from build123d import *

# Parameters (mm, degrees)
F0_W      = 64
F0_H      = 76
F1_DEPTH  = 72
F2_T      = -13
F3_R      = 12.5
F4_DEPTH  = 100
F5_W      = 76
F5_H      = 18
F6_DEPTH  = 56
F8_DEPTH  = 25
F9_W      = 22
F9_H      = 54
F10_DEPTH = 52
F12_DEPTH = 25


with BuildPart() as f1:
    # F0 (on Top) → F1 (new body)
    with BuildSketch(Plane.XY):
        with Locations((32, 38)):
            Rectangle(F0_W, F0_H)
    extrude(amount=F1_DEPTH)

    # F2
    f2_openings = [f1.faces().sort_by_distance(p)[0] for p in [
        (32, 38, 72),
    ]]
    offset(amount=F2_T, openings=f2_openings)

    # F3 (on face) → F4 (cut)
    with BuildSketch(Plane.XZ):
        with Locations((32, 36)):
            Circle(F3_R)
    extrude(amount=-F4_DEPTH, mode=Mode.SUBTRACT)

    # F5 (on face) → F6 (join)
    with BuildSketch(Plane(origin=(0, 0, 0), x_dir=(0, -1, 0), z_dir=(-1, 0, 0))):
        with Locations((-38, 9)):
            Rectangle(F5_W, F5_H)
    extrude(amount=F6_DEPTH)

    # F7 (on face) → F8 (cut)
    with BuildSketch(Plane.XY.offset(18)):
        with BuildLine():
            ThreePointArc((-56, 38), (-44.870058, 64.870058), (-18, 76))
            Line((-18, 76), (-56, 76))
            Line((-56, 76), (-56, 38))
        make_face()
        with BuildLine():
            ThreePointArc((-18, 0), (-44.870058, 11.129942), (-56, 38))
            Line((-56, 38), (-56, 0))
            Line((-56, 0), (-18, 0))
        make_face()
    extrude(amount=-F8_DEPTH, mode=Mode.SUBTRACT)

    # F9 (on face) → F10 (join)
    with BuildSketch(Plane(origin=(0, 0, 0), x_dir=(0, -1, 0), z_dir=(-1, 0, 0))):
        with Locations((-38, 45)):
            Rectangle(F9_W, F9_H)
    extrude(amount=F10_DEPTH)

    # F11 (on face) → F12 (cut)
    with BuildSketch(Plane.XZ.offset(-27)):
        Polygon((-52, 18), (0, 72), (-52, 72), align=None)
    extrude(amount=-F12_DEPTH, mode=Mode.SUBTRACT)


solid = f1.part
Build history of the part. All positions in model axes, mm. A direction names the side the tool comes from. Coordinates: 2 decimals unless noted, no trailing zeros. Write each loop counter-clockwise with the first axis right and the second up, starting at its lowest first coordinate (ties: lowest second). Pieces come first, ordered by that corner, then holes. Notation, with made-up numbers: (4, 13.5) -> (47, 13.5) arc R24 cw to (47, 41.5) -> close; hole circle Ø3 at (-2, 37.25). An arc over 180 degrees is marked (long way). Use CSV: the item, a comma, the result in double quotes. Start each with the question number.
Q1. Pull direction Z, two halves, no side cores. Call faces 1 (the cylindrical face through (22.08, 69.409, 28.394)), 2 (the flat face through (-21, 22, 18)), 3 (the flat face through (42, 0, 27)): released by +Z, released by -Z, zero draft, split by the parting line, or undercut.
Q2. Cut at C-C, the plane y = 58. List the corners of the cut face in (x, z).
Q3. Cut at B-B, the plane z = 40.5. List the corners of the cut face in (x, y).
Q4. Flat gauge pins, fed straight in: pin 1 Ø8 at (y, z) = (61, 43) entering from -X; pin 2 Ø1.5 at (x, z) = (-9.5, 30.5) entering from -Y; pin 3 Ø8 at (y, z) = (17, 14) entering from -X; pin 4 Ø11.5 at (x, z) = (37.5, 38.5) entering from -Y. Where does each tip first touch, or does it go through?
Q5. 3-axis set-ups, long thin cutter, end or side, ignore diameter. For faces 4 (the flat face through (0, 62, 45)), 5 (the flat face through (32, 38, 13)), 6 (the flat face through (64, 37, 35)), 7 (the flat face through (0, 13, 45)): which of +Z, -Z, +X, -X, +Y, -Y reach the whole face in a straight line?
Q6. Cut at D-D, the plane z = 60.5. List the corners of the cut face in (x, y).
Q7. Drill centre lines: probe 1 along Y at (x, z) = (33, 52); probe 2 along Z at (x, y) = (32, 66); probe 3 along X at (y, z) = (54, 36). Where is each one in solid material? Low to high.
Q8. Cut at A-A, the plane x = 32. List the corners of the cut face in (y, z).
Checked values:
1,face 1,"undercut"
1,face 2,"released by +Z"
1,face 3,"zero draft"
2,outline,"(-50.31, 0) -> (64, 0) -> (64, 72) -> (51, 72) -> (51, 13) -> (13, 13) -> (13, 72) -> (0, 72) -> (0, 18) -> (-50.31, 18) -> close"
3,outline,"(-30.33, 27) -> (0, 27) -> (0, 0) -> (20.34, 0) -> (20.34, 13) -> (13, 13) -> (13, 63) -> (20.34, 63) -> (20.34, 76) -> (0, 76) -> (0, 49) -> (-30.33, 49) -> close; (43.66, 0) -> (64, 0) -> (64, 76) -> (43.66, 76) -> (43.66, 63) -> (51, 63) -> (51, 13) -> (43.66, 13) -> close"
4,pin 1,"stops at x = 0"
4,pin 2,"stops at y = 27"
4,pin 3,"stops at x = -51.99"
4,pin 4,"passes through"
5,face 4,"+Z, -X, +Y"
5,face 5,"+Z"
5,face 6,"+Z, -Z, +X, +Y, -Y"
5,face 7,"+Z, -X, -Y"
6,outline,"(-11.07, 27) -> (0, 27) -> (0, 0) -> (64, 0) -> (64, 76) -> (0, 76) -> (0, 49) -> (-11.07, 49) -> close; hole (13, 13) -> (51, 13) -> (51, 63) -> (13, 63) -> close"
7,probe 1,"y = 0 to 13, 63 to 76"
7,probe 2,"z = 0 to 23.5, 48.5 to 72"
7,probe 3,"x = 0 to 13, 51 to 64"
8,outline,"(0, 0) -> (76, 0) -> (76, 23.5) -> (63, 23.5) -> (63, 13) -> (13, 13) -> (13, 23.5) -> (0, 23.5) -> close; (0, 48.5) -> (13, 48.5) -> (13, 72) -> (0, 72) -> close; (63, 48.5) -> (76, 48.5) -> (76, 72) -> (63, 72) -> close"
